from build123d import *

# Parameters (mm, degrees)
F0_R      = 40
F0_R_2    = 2
F0_R_3    = 3.4
F1_DEPTH  = 50
F3_R      = 2.75
F4_DEPTH  = 10
F5_T      = -2.5
F4_FACE_R = 2.75
F6_DEPTH  = 15


with BuildPart() as f1:
    # F0 (on Top) → F1 (new body)
    with BuildSketch(Plane.XY):
        Circle(F0_R)
        with Locations((-16.2671870079, -11.6352321356)):
            Circle(F0_R_2, mode=Mode.SUBTRACT)
        with Locations((11.6352321356, -16.2671870079)):
            Circle(F0_R_2, mode=Mode.SUBTRACT)
        with Locations((-11.6352321356, 16.2671870079)):
            Circle(F0_R_2, mode=Mode.SUBTRACT)
        Circle(F0_R_3, mode=Mode.SUBTRACT)
        with Locations((16.2671870079, 11.6352321356)):
            Circle(F0_R_2, mode=Mode.SUBTRACT)
    extrude(amount=F1_DEPTH)

    # F5
    f5_openings = [f1.faces().sort_by_distance(p)[0] for p in [
        (-38.868629, 0, 0),
    ]]
    offset(amount=F5_T, openings=f5_openings)


with BuildPart() as f4:
    # F3 (on face) → F4 (new body)
    with BuildSketch(Plane.XY.offset(50)):
        with Locations((-11.6352321356, 16.2671870079)):
            Circle(F3_R)
    extrude(amount=-F4_DEPTH)


with BuildPart() as f4b:
    # F3 (on face) → F4, piece 2 (new body)
    with BuildSketch(Plane.XY.offset(50)):
        with Locations((16.2671870079, 11.6352321356)):
            Circle(F3_R)
    extrude(amount=-F4_DEPTH)


with BuildPart() as f4c:
    # F3 (on face) → F4, piece 3 (new body)
    with BuildSketch(Plane.XY.offset(50)):
        with Locations((11.6352321356, -16.2671870079)):
            Circle(F3_R)
    extrude(amount=-F4_DEPTH)


with BuildPart() as f4d:
    # F3 (on face) → F4, piece 4 (new body)
    with BuildSketch(Plane.XY.offset(50)):
        with Locations((-16.2671870079, -11.6352321356)):
            Circle(F3_R)
    extrude(amount=-F4_DEPTH)


with BuildPart() as f6_tool:
    # F4_face (on face) → F6 (new body)
    with BuildSketch(Plane(origin=(-11.6352321356, 16.2671870079, 50), x_dir=(1, 0, 0), z_dir=(0, 0, 1))):
        Circle(F4_FACE_R)
        with Locations((23.2704642711, -32.5343740159)):
            Circle(F4_FACE_R)
        with Locations((27.9024191435, -4.6319548724)):
            Circle(F4_FACE_R)
        with Locations((-4.6319548724, -27.9024191435)):
            Circle(F4_FACE_R)
    extrude(amount=-F6_DEPTH)


with BuildPart() as f1_1:
    add(f1.part)

    # F6: cut by f6_tool
    add(f6_tool.part, mode=Mode.SUBTRACT)


with BuildPart() as f4_1:
    add(f4.part)

    # F6: cut by f6_tool
    add(f6_tool.part, mode=Mode.SUBTRACT)


with BuildPart() as f4b_1:
    add(f4b.part)

    # F6: cut by f6_tool
    add(f6_tool.part, mode=Mode.SUBTRACT)


with BuildPart() as f4c_1:
    add(f4c.part)

    # F6: cut by f6_tool
    add(f6_tool.part, mode=Mode.SUBTRACT)


with BuildPart() as f4d_1:
    add(f4d.part)

    # F6: cut by f6_tool
    add(f6_tool.part, mode=Mode.SUBTRACT)


solid = f1_1.part
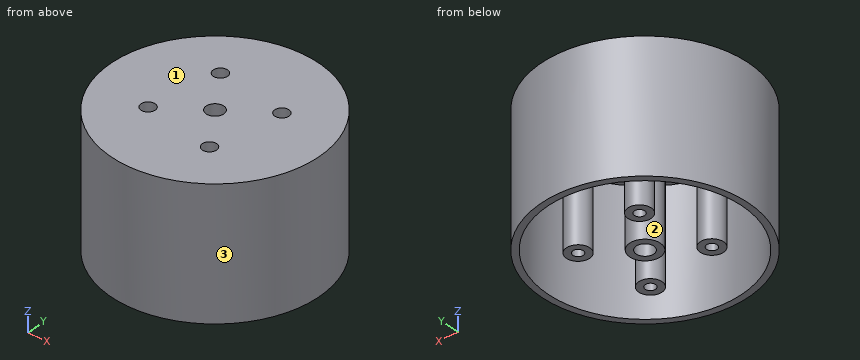
Check sheet for the modelled part. Datum: model origin and axes. Units: mm. Face numbers are marked on the shaded views. Round coordinates to 2 decimals unless told otherwise and drop trailing zeros. Order: outer loops, then holes, each group sorted by start corner. A loop starts at its lowest first (then second) coordinate and runs counter-clockwise, first axis right, second up.
Q1. Cross-section at B-B, the plane z = 37.5. Give the number of separate pieces and of enclosed holes in the cut face, plus the area to 3 significant figures.
Filled sheet:
separate pieces: 6
enclosed holes: 6
area: 841 mm2
Q2. Cross-section at D-D, the plane y = -22. Enter the section's corners in (x, z).
Filled sheet:
outline: (-33.41, 0) - (-30.37, 0) - (-30.37, 47.5) - (30.37, 47.5) - (30.37, 0) - (33.41, 0) - (33.41, 50) - (-33.41, 50) - close
Q3. Depth check by flat-ended pin: P1, Ø10, axis at y = -30, z = 28.5, coming from the +X side (3 decimals); P2, Ø10, axis at x = -0.5, z = 23, coming from the +Y side; P3, Ø2.5, axis at x = 11.64, y = -16.27, coming from the -Z side; P4, Ø6, axis at y = -13, z = 35.5, coming from the +X side. Enter the tip coordinate at first touch or a pass-through.
Filled sheet:
P1: stops at x = 31.225
P2: stops at y = 40
P3: passes through
P4: stops at x = 38.73
Q4. Draft check along X on the marked faces 1, 2 and 3. Enter one of: pulls with the +X half, pulls with the -X half, needs draft (parallel to the pull), parting line crosses it, or undercut.
Filled sheet:
face 1: needs draft
face 2: undercut
face 3: parting line crosses it
Q5. Cross-section at A-A, the plane x = 0. Enter the section's corners in (y, z), plus the area to 3 significant figures.
Filled sheet:
outline: (-40, 0) - (-37.5, 0) - (-37.5, 47.5) - (-5.9, 47.5) - (-5.9, 0) - (-3.4, 0) - (-3.4, 50) - (-40, 50) - close; (3.4, 0) - (5.9, 0) - (5.9, 47.5) - (37.5, 47.5) - (37.5, 0) - (40, 0) - (40, 50) - (3.4, 50) - close
area: 658 mm2
Q6. Scan lines: L1, parallel to Y at x = 0, z = 32.5; L2, parallel to X at y = 4, z = 39; L3, parallel to X at y = -2, z = 12. Record each from-to range of solid material in increasing order.
Filled sheet:
L1: y = -40 to -37.5, -5.9 to -3.4, 3.4 to 5.9, 37.5 to 40
L2: x = -39.8 to -37.29, -4.34 to 4.34, 37.29 to 39.8
L3: x = -39.95 to -37.45, -5.55 to -2.75, 2.75 to 5.55, 37.45 to 39.95
